```python
from build123d import *

# Parameters (mm, degrees)
PAD_DEPTH    = 1200
SKETCH001_R  = 25
POCKET_DEPTH = 11


with BuildPart() as part:
    # Sketch → Pad (new body)
    with BuildSketch(Plane.XZ):
        Polygon((-71.120202, 50.807465), (23.879798, 50.807465), (23.879798, -89.192535), (-71.120202, -89.192535), (-71.120202, -94.192535), (28.879798, -94.192535), (28.879798, 55.807465), (-71.120202, 55.807465), align=None)
    extrude(amount=PAD_DEPTH)

    # Sketch001 (on DatumPlane) → Pocket (cut)
    with BuildSketch(Plane(origin=(28.879798, 0, 0), x_dir=(0, 0, 1), z_dir=(1, 0, 0))):
        with Locations((-19.580029, 932.952332)):
            Circle(SKETCH001_R)
        with Locations((-24.085371, 375.785522)):
            Circle(SKETCH001_R)
    extrude(amount=-POCKET_DEPTH, mode=Mode.SUBTRACT)


solid = part.part
```
Verification items for the finished model (mm, model axes). A direction names the side the tool comes from. Round coordinates to 2 decimals unless told otherwise and drop trailing zeros. Order: outer loops, then holes, each group sorted by start corner. A loop starts at its lowest first (then second) coordinate and runs counter-clockwise, first axis right, second up.
1) Draft check along Y on faces 3 (the cylindrical face through (26.41, -351.38, -29.5)), 4 (the flat face through (28.88, -592, -20)), 5 (the flat face through (27, -1200, -19)). Enter one of: +Y half, -Y half, draft (parallel to the pull), parting line (faces both ways), or undercut.
Geometry says:
face 3: undercut
face 4: draft
face 5: -Y half
2) Cross-section at D-D, the plane y = -390.5. Record the cut outline in (x, z).
Geometry says:
outline: (-71.12, -94.19) - (28.88, -94.19) - (28.88, -44.3) - (23.88, -44.3) - (23.88, -89.19) - (-71.12, -89.19) - close; (-71.12, 50.81) - (23.88, 50.81) - (23.88, -3.87) - (28.88, -3.87) - (28.88, 55.81) - (-71.12, 55.81) - close
3) Tool access check on faces 1 (the flat face through (23.88, -592, -18)), 2 (the flat face through (-22, -592, -94.193)). Record the directions out of +Z, -Z, +X, -X, +Y, -Y that give a thin tool (end or side, any length) a straight path to the whole face; none if there is none.
Geometry says:
face 1: -X, +Y, -Y
face 2: -Z, +X, -X, +Y, -Y
4) Cross-section at B-B, the plane y = -990. Record the cut outline in (x, z), plus the area to 3 significant figures.
Geometry says:
outline: (-71.12, -94.19) - (28.88, -94.19) - (28.88, 55.81) - (-71.12, 55.81) - (-71.12, 50.81) - (23.88, 50.81) - (23.88, -89.19) - (-71.12, -89.19) - close
area: 1,700 mm2
5) Cross-section at C-C, the plane z = -31.5. Record the cut outline in (x, y), plus the area to 3 significant figures.
Geometry says:
outline: (23.88, -1200) - (28.88, -1200) - (28.88, -954.93) - (23.88, -954.93) - close; (23.88, -910.98) - (28.88, -910.98) - (28.88, -399.66) - (23.88, -399.66) - close; (23.88, -351.91) - (28.88, -351.91) - (28.88, 0) - (23.88, 0) - close
area: 5,540 mm2
6) Material ranges on line 1 (Z direction, x = 12, y = -1034); line 2 (X direction, y = -780, z = -12.5), recorded low to high.
Geometry says:
line 1: z = -94.19 to -89.19, 50.81 to 55.81
line 2: x = 23.88 to 28.88
7) Cross-section at A-A, the plane x = -5.5. Record the cut outline in (y, z).
Geometry says:
outline: (-1200, -94.19) - (0, -94.19) - (0, -89.19) - (-1200, -89.19) - close; (-1200, 50.81) - (0, 50.81) - (0, 55.81) - (-1200, 55.81) - close
